Build history of the part. All positions in model axes, mm. Round coordinates to 2 decimals unless told otherwise and drop trailing zeros. Write each loop counter-clockwise with the first axis right and the second up, starting at its lowest first coordinate (ties: lowest second). Pieces come first, ordered by that corner, then holes. Notation, with made-up numbers: M 25.25,8 L 77.25,8 A29 ccw 77.25,45 Z; hole C 33,88 d1. An arc over 180 degrees is marked long. Write item = value, one per line.
Autodesk Inventor part; units mm, degrees
ref_plane "YZ Plane" through (0, 0, 0) normal (1, 0, 0) x (0, 1, 0)
ref_plane "XZ Plane" through (0, 0, 0) normal (0, 1, 0) x (-1, 0, 0)
ref_plane "XY Plane" through (0, 0, 0) normal (0, 0, 1) x (1, 0, 0)
sketch "Sketch1" plane through (0, 0, 0) normal (0, 0, 1) x (1, 0, 0)
  line L0 (0, 356.108) -> (0, -314.198)
  line L1 (-609.6, 0) -> (457.2, 0)
  line L2 (304.8, -218.44) -> (-457.2, -218.44)
  line L3 (-457.2, -218.44) -> (-457.2, 260.35)
  line L4 (-457.2, 260.35) -> (304.8, 260.35)
  line L5 (304.8, 260.35) -> (304.8, -218.44)
  line L6 (260.35, -135.89) -> (-260.35, -135.89) construction
  line L7 (-260.35, -135.89) -> (-260.35, 194.31) construction
  line L8 (-260.35, 194.31) -> (260.35, 194.31) construction
  line L9 (260.35, 194.31) -> (260.35, -135.89) construction
  line L10 (260.35, -135.89) -> (-260.35, 194.31) construction
  line L11 (-260.35, -135.89) -> (260.35, 194.31) construction
  line L12 (292.1, -142.24) -> (-444.5, -142.24) construction
  line L13 (-444.5, -142.24) -> (-444.5, 142.24) construction
  line L14 (-444.5, 142.24) -> (292.1, 142.24) construction
  line L15 (292.1, 142.24) -> (292.1, -142.24) construction
  line L16 (215.9, -123.19) -> (-215.9, -123.19) construction
  line L17 (-215.9, -123.19) -> (-215.9, 181.61) construction
  line L18 (-215.9, 181.61) -> (215.9, 181.61) construction
  line L19 (215.9, 181.61) -> (215.9, -123.19) construction
  line L20 (215.9, -123.19) -> (-215.9, 181.61) construction
  line L21 (-215.9, -123.19) -> (215.9, 181.61) construction
  line L22 (76.2, -135.89) -> (-76.2, -135.89) construction
  line L23 (-76.2, -135.89) -> (-76.2, -167.64) construction
  line L24 (-76.2, -167.64) -> (76.2, -167.64) construction
  line L25 (76.2, -167.64) -> (76.2, -135.89) construction
  line L26 (76.2, -135.89) -> (-76.2, -167.64) construction
  line L27 (-76.2, -135.89) -> (76.2, -167.64) construction
  point P0 (0, 0)
  point P1 (0, 29.21)
  point P2 (0, 0)
  point P3 (228.6, -199.39)
  point P4 (-381, -199.39)
  point P5 (-76.2, -199.39)
  point P6 (0, -151.765)
  point P7 (-381, 241.3)
  point P8 (-76.2, 241.3)
  point P9 (228.6, 241.3)
  dimension "d1" = 762
  dimension "d2" = 520.7
  dimension "d3" = 330.2
  dimension "d4" = 82.55
  dimension "d5" = 736.6
  dimension "d6" = 76.2
  dimension "d28" = 431.8
  dimension "d29" = 304.8
  dimension "d38" = 304.8
  dimension "d39" = 260.35
  dimension "d40" = 292.1
  dimension "d41" = 19.05
  dimension "d42" = 76.2
  dimension "d43" = 76.2
  dimension "d44" = 304.8
  dimension "d46" = 304.8
  dimension "d47" = 50.8
  dimension "d48" = 31.75
  dimension "d49" = 152.4
  dimension "d60" = 142.24
  dimension "d61" = 218.44
  dimension "d64" = 19.05
extrude "Extrusion1" add sketch "Sketch1" against normal blind 6.35
hole "Hole1" at (-260.35, 194.31, 0) at (-260.35, -135.89, 0) at (260.35, -135.89, 0) at (260.35, 194.31, 0) direction (0, 0, -1) diameter 9.525 end through all
hole "Hole2" at (-444.5, -142.24, 0) at (-444.5, 142.24, 0) at (292.1, 142.24, 0) at (292.1, -142.24, 0) at (-381, -199.39, 0) at (-76.2, -199.39, 0) at (228.6, -199.39, 0) at (-381, 241.3, 0) at (-76.2, 241.3, 0) at (228.6, 241.3, 0) direction (0, 0, -1) diameter 11.43 end through all
sketch "Sketch2" plane through (0, 0, 0) normal (0, 0, 1) x (1, 0, 0)
  line L0 (-457.2, -218.44) -> (-457.2, 260.35)
  line L1 (-457.2, -218.44) -> (-421.64, -218.44)
  line L2 (-421.64, -218.44) -> (-421.64, -177.8)
  line L3 (-421.64, -177.8) -> (-457.2, -177.8)
  line L4 (-457.2, -177.8) -> (-457.2, -218.44)
  line L5 (304.8, -218.44) -> (-457.2, -218.44)
  line L6 (304.8, -218.44) -> (269.24, -218.44)
  line L7 (269.24, -218.44) -> (269.24, -177.8)
  line L8 (269.24, -177.8) -> (304.8, -177.8)
  line L9 (304.8, -177.8) -> (304.8, -218.44)
  line L10 (-457.2, 219.71) -> (-421.64, 219.71)
  line L11 (-421.64, 219.71) -> (-421.64, 260.35)
  line L12 (-457.2, 260.35) -> (304.8, 260.35)
  line L13 (269.24, 260.35) -> (269.24, 219.71)
  line L14 (269.24, 219.71) -> (304.8, 219.71)
  line L15 (304.8, 260.35) -> (304.8, -218.44)
  point P0 (0, 0)
  dimension "d24" = 35.56
  dimension "d37" = 40.64
  dimension "d62" = 35.56
  dimension "d63" = 40.64
extrude "Extrusion2" cut sketch "Sketch2" against normal blind 6.35 contours L0 L3 L2 L1 | L0 L12 L11 L10 | L7 L8 L9 L5 | L12 L15 L14 L13
fillet "Fillet1" radius 6.35 8 edges at (269.24, -218.44, -3.175) (304.8, -177.8, -3.175) (-421.64, -218.44, -3.175) (-457.2, -177.8, -3.175) (-457.2, 219.71, -3.175) (-421.64, 260.35, -3.175) (269.24, 260.35, -3.175) (304.8, 219.71, -3.175)
hole "Hole3" at (-215.9, 181.61, 0) at (215.9, 181.61, 0) at (215.9, -123.19, 0) at (-215.9, -123.19, 0) direction (0, 0, -1) diameter 38.1 end through all
hole "Hole4" at (-76.2, -135.89, 0) at (-76.2, -167.64, 0) direction (0, 0, -1) diameter 3.1242 depth 25.4 tip angle 118
pattern_linear "Rectangular Pattern1" count 4 spacing 50.8 along (1, 0, 0) of "Hole4"
sketch "Sketch3" plane through (0, 0, 0) normal (0, 0, 1) x (1, 0, 0)
  line L0 (0, 356.108) -> (0, -314.198)
  line L1 (-609.6, 0) -> (457.2, 0)
  line L2 (25.4, 199.39) -> (-25.4, 199.39)
  line L3 (-25.4, 199.39) -> (-25.4, 224.79)
  line L4 (-25.4, 224.79) -> (25.4, 224.79)
  line L5 (25.4, 224.79) -> (25.4, 199.39)
  line L6 (25.4, 199.39) -> (-25.4, 224.79) construction
  line L7 (-25.4, 199.39) -> (25.4, 224.79) construction
  line L8 (-415.29, 260.35) -> (262.89, 260.35)
  line L9 (-355.6, 199.39) -> (-406.4, 199.39)
  line L10 (-406.4, 199.39) -> (-406.4, 224.79)
  line L11 (-406.4, 224.79) -> (-355.6, 224.79)
  line L12 (-355.6, 224.79) -> (-355.6, 199.39)
  line L13 (-355.6, 199.39) -> (-406.4, 224.79) construction
  line L14 (-406.4, 199.39) -> (-355.6, 224.79) construction
  line L15 (-25.4, 224.79) -> (-76.2, 224.79)
  line L16 (-76.2, 224.79) -> (-76.2, 199.39)
  line L17 (-76.2, 199.39) -> (-25.4, 199.39)
  line L18 (-25.4, 199.39) -> (-25.4, 224.79)
  point P0 (0, 0)
  point P1 (0, 212.09)
  point P2 (-381, 212.09)
  point P3 (-381, 212.09)
  point P4 (0, 212.09)
  point P5 (-342.9, 212.09)
  point P6 (-419.1, 212.09)
  point P7 (38.1, 224.79)
  point P8 (-38.1, 224.79)
  point P9 (0, 212.09)
  point P10 (-381, 212.09)
  point P11 (-196.85, 224.79)
  point P12 (-215.9, 181.61)
  point P13 (-209.55, 224.79)
  point P14 (-222.25, 224.79)
  point P15 (-234.95, 224.79)
  dimension "d65" = 35.56
  dimension "d66" = 50.8
  dimension "d67" = 25.4
  dimension "d68" = 381
  dimension "d69" = 50.8
  dimension "d91" = 38.1
  dimension "d92" = 38.1
  dimension "d95" = 12.7
  dimension "d96" = 38.1
  dimension "d97" = 38.1
  dimension "d98" = 25.4
  dimension "d99" = 50.8
  dimension "d100" = 19.05
  dimension "d103" = 12.7
extrude "Extrusion3" cut sketch "Sketch3" against normal through all
fillet "Fillet2" radius 3.175 8 edges at (-406.4, 224.79, -3.175) (-355.6, 224.79, -3.175) (-355.6, 199.39, -3.175) (-406.4, 199.39, -3.175) (25.4, 224.79, -3.175) (25.4, 199.39, -3.175) (-76.2, 224.79, -3.175) (-76.2, 199.39, -3.175)
fillet "Fillet3" radius 3.175 4 edges at (-421.64, -177.8, -3.175) (269.24, -177.8, -3.175) (269.24, 219.71, -3.175) (-421.64, 219.71, -3.175)
sketch "Sketch4" plane through (0, 0, 0) normal (0, 0, 1) x (1, 0, 0)
  line L0 (-444.5, -142.24) -> (-444.5, 142.24) construction
  line L1 (292.1, 142.24) -> (292.1, -142.24) construction
  circle A0 centre (292.1, -142.24) radius 5.715
  circle A1 centre (-381, 241.3) radius 5.715 construction
  circle A2 centre (228.6, 241.3) radius 5.715 construction
  line L2 (-381, 241.3) -> (228.6, 241.3) construction
  line L3 (-406.4, -161.29) -> (-304.8, -161.29) construction
  line L4 (-304.8, -161.29) -> (-304.8, -85.09) construction
  line L5 (-304.8, -85.09) -> (-406.4, -85.09) construction
  line L6 (-406.4, -85.09) -> (-406.4, -161.29) construction
  point P0 (0, 0)
  point P1 (-444.5, -66.04)
  point P2 (-444.5, 66.04)
  point P3 (292.1, 66.04)
  point P4 (292.1, -66.04)
  point P5 (292.1, -66.04)
  point P6 (-304.8, 241.3)
  point P7 (152.4, 241.3)
  point P8 (-406.4, -123.19)
  point P9 (-304.8, -123.19)
  point P10 (-381, -199.39)
  point P11 (-355.6, -85.09)
  point P12 (-355.6, -161.29)
  point P13 (-419.1, 212.09)
  point P14 (-342.9, 212.09)
  point P15 (-38.1, 224.79)
  point P16 (38.1, 224.79)
  dimension "d74" = 76.2
  dimension "d75" = 76.2
  dimension "d76" = 76.2
  dimension "d77" = 76.2
  dimension "d85" = 76.2
  dimension "d86" = 76.2
  dimension "d87" = 101.6
  dimension "d88" = 76.2
  dimension "d89" = 38.1
  dimension "d90" = 38.1
hole "Hole5" at (-444.5, 66.04, 0) at (-444.5, -66.04, 0) at (292.1, 66.04, 0) at (292.1, -66.04, 0) at (-406.4, -85.09, 0) at (-355.6, -85.09, 0) at (-304.8, -85.09, 0) at (-304.8, -123.19, 0) at (-304.8, -161.29, 0) at (-355.6, -161.29, 0) at (-406.4, -161.29, 0) at (-406.4, -123.19, 0) at (-419.1, 212.09, 0) at (-342.9, 212.09, 0) at (38.1, 224.79, 0) direction (0, 0, -1) diameter 3.1242 end through all
hole "Hole6" at (-234.95, 224.79, 0) at (-222.25, 224.79, 0) at (-209.55, 224.79, 0) at (-196.85, 224.79, 0) direction (0, 0, -1) diameter 7.9375 end through all
properties material "ACETAL COPOLYMER, BLACK"
1. Probe probe 1 along Y at (x, z) = (260.35, -2); probe 2 along Y at (x, z) = (215.9, -3.5); probe 3 along Y at (x, z) = (-25.4, -4). List the from-to ranges inside material, lowest first.
Responses:
probe_1 = -218.44 to -140.65, -131.13 to 189.55, 199.07 to 260.35
probe_2 = -218.44 to -142.24, -104.14 to 162.56, 200.66 to 260.35
probe_3 = -218.44 to -169.2, -166.08 to -137.45, -134.33 to 199.39, 224.79 to 260.35
2. Band-saw the part on A-A (x = -16). List the corners of the cut face in (y, z), plus the area to 3 significant figures.
Responses:
outline = M -218.44,-6.35 L 199.39,-6.35 L 199.39,0 L -218.44,0 Z; M 224.79,-6.35 L 260.35,-6.35 L 260.35,0 L 224.79,0 Z
area = 2,880 mm²
3. Band-saw the part on B-B (z = -2.5). Count the separate pieces of the cut face and the enclosed holes in it, plus the area to 3 significant figures.
Responses:
separate_pieces = 1
enclosed_holes = 47
area = 349,000 mm²
4. Flat gauge pins, fed straight in: pin 1 (5 mm diameter, centred on x = -419.1, y = 212.09, fed in from +Z); pin 2 (6.5 mm diameter, centred on x = -234.95, y = 224.79, fed in from +Z). Where does each tip first touch, or does it go through?
Responses:
pin_1 = 0
pin_2 = through
5. Mould opens along X. For faces 1 (the face through (-199, -131.98, -3.22)), 2 (the face through (-82, 24, 0)) say: pulls with the +X half, pulls with the -X half, needs draft (parallel to the pull), parting line crosses it, or undercut.
Responses:
face_1 = undercut
face_2 = needs draft
